```python
from build123d import *

# Parameters (mm, degrees)
SKETCH2_W           = 5.5
SKETCH2_H           = 3.17
BOSS_EXTRUDE1_DEPTH = 25
SKETCH3_R           = 1.4
CUT_EXTRUDE1_DEPTH  = 27.583939305
SKETCH6_W           = 3.5
SKETCH6_H           = 3
BOSS_EXTRUDE2_DEPTH = 15
FILLET2_R           = 1


with BuildPart() as part:
    # Sketch1 → Revolve1 (revolve)
    with BuildSketch(Plane.XY):
        Polygon((0, 0), (25, 0), (10, -10), (0, -10), align=None)
    revolve(axis=Axis((0, 0, 0), (0, -1, 0)))

    # Sketch2 → Boss-Extrude1 (add)
    with BuildSketch(Plane.XZ.offset(10)):
        with Locations((-0.00136169, 0.001060695)):
            Rectangle(SKETCH2_W, SKETCH2_H)
    extrude(amount=BOSS_EXTRUDE1_DEPTH)

    # Sketch3 → Cut-Extrude1 (cut, through all)
    with BuildSketch(Plane(origin=(0, 0, -1.583939305), x_dir=(-1, 0, 0), z_dir=(0, 0, -1))):
        with Locations((0, -32.128448622)):
            Circle(SKETCH3_R)
    extrude(amount=-CUT_EXTRUDE1_DEPTH, mode=Mode.SUBTRACT)

    # Sketch6 → Boss-Extrude2 (add)
    with BuildSketch(Plane.XZ.offset(10)):
        with Locations((-0.00136169, -5.083939305)):
            Rectangle(SKETCH6_W, SKETCH6_H)
        with Locations((-0.00136169, 5.086060695)):
            Rectangle(SKETCH6_W, SKETCH6_H)
    extrude(amount=BOSS_EXTRUDE2_DEPTH)

    # Fillet2
    fillet2_edges = [part.edges().sort_by_distance(p)[0] for p in [
        (-25, 0, 0),
    ]]
    fillet(fillet2_edges, radius=FILLET2_R)


solid = part.part
```
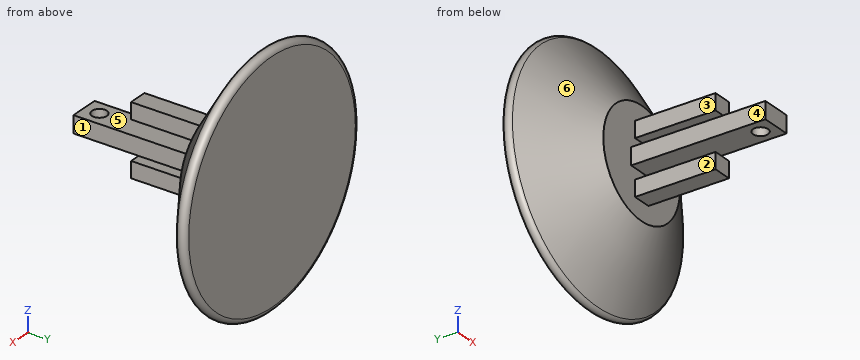
Model file for the job. Use its own axes, mm. Face numbers are marked on the shaded views. A direction names the side the tool comes from. Give positions to 0.01 mm unless a question says otherwise; leave off trailing zeros. Write each loop counter-clockwise with the first axis right and the second up, starting at its lowest first coordinate (ties: lowest second). Pieces come first, ordered by that corner, then holes. Notation, with made-up numbers: M 67,-14.75 L 92,-14.75 A31 ccw 92,16.25 Z; hole C 82.5,63 d9. An arc over 180 degrees is marked long. Use a Markdown table: item, result.
1) Cut at B-B (y = -11.5). List the corners of the cut face in (x, z).
Responses:
| item | result |
|---|---|
| outline | M -2.75,-1.58 L 2.75,-1.58 L 2.75,1.59 L -2.75,1.59 Z; M -1.75,-6.58 L 1.75,-6.58 L 1.75,-3.58 L -1.75,-3.58 Z; M -1.75,3.59 L 1.75,3.59 L 1.75,6.59 L -1.75,6.59 Z |
2) Pin check, flat tips, straight feed: pin 1 (2 mm diameter, centred on y = -21, z = -9, fed in from -X); pin 2 (1.5 mm diameter, centred on y = -18, z = -4.5, fed in from -X); pin 3 (3.5 mm diameter, centred on x = 0, z = 4.5, fed in from -Y); pin 4 (1 mm diameter, centred on y = -28, z = -0.5, fed in from -X). Stop position of each tip, or through.
Responses:
| item | result |
|---|---|
| pin 1 | passes through |
| pin 2 | stops at x = -1.75 |
| pin 3 | stops at y = -25 |
| pin 4 | stops at x = -2.75 |
3) Pull direction Z, two halves, no side cores. Call the marked faces 4, 5 and 6: +Z half, -Z half, draft (parallel to the pull), parting line (faces both ways), or undercut.
Responses:
| item | result |
|---|---|
| face 4 | draft |
| face 5 | undercut |
| face 6 | parting line |
4) Cut at C-C (z = 0). List the corners of the cut face in (x, y), and give its area (3 significant figures).
Responses:
| item | result |
|---|---|
| outline | M -22.25,-1.83 L -10,-10 L -2.75,-10 L -2.75,-35 L 2.75,-35 L 2.75,-10 L 10,-10 L 22.25,-1.83 A1 ccw 21.7,0 L -21.7,0 A1 ccw Z; hole C 0,-32.13 d2.8 |
| area | 477 mm2 |
5) Drill centre lines: line 1 (Y direction, x = 0, z = -0.3); line 2 (X direction, y = -15, z = -1); line 3 (X direction, y = -23.5, z = -4.5). Where is each one in solid material? Low to high. Write a range as from..to.
Responses:
| item | result |
|---|---|
| line 1 | y = -35..-33.53, -30.73..0 |
| line 2 | x = -2.75..2.75 |
| line 3 | x = -1.75..1.75 |
6) Tool access for the marked faces 1, 2 and 3: list every direction of +Z, -Z, +X, -X, +Y, -Y with a clear straight run to the whole face (end or side of a thin tool).
Responses:
| item | result |
|---|---|
| face 1 | +Z, -Z, +X, -Y |
| face 2 | -Z, -X, -Y |
| face 3 | +Z, -X, -Y |
7) Cut at D-D (y = -28). List the corners of the cut face in (x, z), and give its area (3 significant figures).
Responses:
| item | result |
|---|---|
| outline | M -2.75,-1.58 L 2.75,-1.58 L 2.75,1.59 L -2.75,1.59 Z |
| area | 17.4 mm2 |
8) Cut at A-A (x = 0). List the corners of the cut face in (y, z).
Responses:
| item | result |
|---|---|
| outline | M -35,-1.58 L -33.53,-1.58 L -33.53,1.59 L -35,1.59 Z; M -30.73,-1.58 L -10,-1.58 L -10,-3.58 L -25,-3.58 L -25,-6.58 L -10,-6.58 L -10,-10 L -1.83,-22.25 A1 ccw 0,-21.7 L 0,21.7 A1 ccw -1.83,22.25 L -10,10 L -10,6.59 L -25,6.59 L -25,3.59 L -10,3.59 L -10,1.59 L -30.73,1.59 Z |
